Geometry check sheet. Reference: the model listing, model coordinates, mm. A direction names the side the tool comes from. Coordinates: 2 decimals unless noted, no trailing zeros. Loops run counter-clockwise (first coordinate to the right, second up) from the corner with the lowest first, then second, coordinate; pieces in that order, holes last. Notation, with made-up numbers: (67, 39.25) - (109, 39.25) arc R11 cw to (109, 53.25) - close; hole circle Ø10 at (-7.5, 76.5). An arc over 180 degrees is marked (long way). Write each question's results on one line, items separated by ' | '. Start each with the question number.
(1) Sectioned sample at C-C (x = 18). Enter the section's corners in (y, z).
(2) Material ranges on probe 1 along Y at (x, z) = (0, 3.9); probe 2 along Z at (x, y) = (1, 12.5); probe 3 along Y at (x, z) = (0, 1.4), recorded low to high.
(3) Mould release check, pull along X, two halves, no side actions. Record for faces 1 (the face through (-18.895, -14.488, 1.479)), 2 (the face through (5, 0, 27)), 3 (the face through (-9.476, -11.94, 1.521)): pulls with the +X half, pulls with the -X half, needs draft (parallel to the pull), parting line crosses it, or undercut.
(4) Sectioned sample at A-A (x = 11). Enter the section's corners in (y, z), plus the area to 3 significant figures.
(5) Access from +Z, -Z, +X, -X, +Y, -Y to the whole of each face (thin tool, end or side, straight path). Record for faces 4 (the face through (-0.534, -4.065, 2.535)), 5 (the face through (0, -1, 9)), 6 (the face through (0.158, 16.737, 1.521)).
(6) Sectioned sample at B-B (z = 20.5). Enter the section's corners in (x, y).
(7) Go/stop test with flat-tipped pins: pin 1 Ø1.6 at (x, y) = (-15.64, -0.54) entering from -Z; pin 2 Ø4 at (x, y) = (10.68, 11.44) entering from +Z; pin 3 Ø4 at (x, y) = (-11.44, 10.68) entering from -Z; pin 4 Ø1 at (x, z) = (0, 18.5) entering from -Y. Record where each tip stops, or that it passes through.
from build123d import *

# Parameters (mm, degrees)
ESQUISSE1_R             = 23.81
BOSS_EXTRU_1_DEPTH      = 3
ESQUISSE2_R             = 12
BOSS_EXTRU_2_DEPTH      = 24
ESQUISSE3_R             = 1.3
ENL_V_MAT_EXTRU_1_DEPTH = 24
ESQUISSE4_R             = 4.1
ENL_V_MAT_EXTRU_2_DEPTH = 18
ESQUISSE5_R             = 0.4
ENL_V_MAT_EXTRU_3_DEPTH = 10
ENL_V_START             = -5
ESQUISSE6_R             = 4.1
ENL_V_MAT_EXTRU_4_DEPTH = 5


with BuildPart() as part:
    # Esquisse1 → Boss.-Extru.1 (new body)
    with BuildSketch(Plane.XY):
        Circle(ESQUISSE1_R)
    extrude(amount=BOSS_EXTRU_1_DEPTH)

    # Esquisse2 → Boss.-Extru.2 (add)
    with BuildSketch(Plane.XY.offset(3)):
        Circle(ESQUISSE2_R)
    extrude(amount=BOSS_EXTRU_2_DEPTH)

    # Esquisse3 → Enl_v. mat.-Extru.1 (cut)
    with BuildSketch(Plane.XY.offset(3)):
        with Locations((-11.442120986, 10.677095455)):
            Circle(ESQUISSE3_R)
        with Locations((-0.540954741, 15.64064794)):
            Circle(ESQUISSE3_R)
        with Locations((10.677095455, 11.442120986)):
            Circle(ESQUISSE3_R)
        with Locations((15.64064794, 0.540954741)):
            Circle(ESQUISSE3_R)
        with Locations((11.442120986, -10.677095455)):
            Circle(ESQUISSE3_R)
        with Locations((0.540954741, -15.64064794)):
            Circle(ESQUISSE3_R)
        with Locations((-10.677095455, -11.442120986)):
            Circle(ESQUISSE3_R)
        with Locations((-15.64064794, -0.540954741)):
            Circle(ESQUISSE3_R)
    extrude(amount=-ENL_V_MAT_EXTRU_1_DEPTH, mode=Mode.SUBTRACT)

    # Esquisse4 → Enl_v. mat.-Extru.2 (cut)
    with BuildSketch(Plane.XY.offset(27)):
        Circle(ESQUISSE4_R)
    extrude(amount=-ENL_V_MAT_EXTRU_2_DEPTH, mode=Mode.SUBTRACT)

    # Esquisse5 → Enl_v. mat.-Extru.3 (cut)
    with BuildSketch(Plane(origin=(0, 0, 0), x_dir=(-1, 0, 0), z_dir=(0, 0, -1))):
        Circle(ESQUISSE5_R)
    extrude(amount=-ENL_V_MAT_EXTRU_3_DEPTH, mode=Mode.SUBTRACT)

    # Esquisse6 → Enl_v. mat.-Extru.4 (cut)
    with BuildSketch(Plane(origin=(0, 0, 0), x_dir=(-1, 0, 0), z_dir=(0, 0, -1)).offset(ENL_V_START)):
        with Locations(Location((0, 0, 0), (0, 0, 180))):
            Circle(ESQUISSE6_R)
    extrude(amount=ENL_V_MAT_EXTRU_4_DEPTH, mode=Mode.SUBTRACT)


solid = part.part
Outcome:
1) outline: (-15.59, 0) - (15.59, 0) - (15.59, 3) - (-15.59, 3) - close
2) probe 1: y = -12 to -4.1, 4.1 to 12 | probe 2: z = 0 to 3 | probe 3: y = -23.81 to -16.82, -14.46 to -4.1, 4.1 to 14.46, 16.82 to 23.81
3) face 1: parting line crosses it | face 2: needs draft | face 3: undercut
4) outline: (-21.12, 0) - (-11.9, 0) - (-11.9, 3) - (-21.12, 3) - close; (-9.45, 0) - (10.18, 0) - (10.18, 3) - (4.8, 3) - (4.8, 27) - (-4.8, 27) - (-4.8, 3) - (-9.45, 3) - close; (12.7, 0) - (21.12, 0) - (21.12, 3) - (12.7, 3) - close | area: 342 mm2
5) face 4: -Z | face 5: +Z | face 6: +Z, -Z
6) outline: circle Ø24 at (0, 0); hole circle Ø8.2 at (0, 0)
7) pin 1: passes through | pin 2: stops at z = 3 | pin 3: stops at z = 0 | pin 4: stops at y = -12
